For this review, use the dimensioned drawing (mm, ordinates from the lowest corner) and the shaded views. A direction names the side the tool comes from. Round coordinates to 2 decimals unless told otherwise and drop trailing zeros. Order: outer loops, then holes, each group sorted by start corner. A loop starts at its lowest first (then second) coordinate and runs counter-clockwise, first axis right, second up. Notation, with made-up numbers: (-6.75, 56) -> (39.25, 56) arc R19 cw to (39.25, 92) -> close; hole circle Ø11 at (64, -31). An arc over 180 degrees is marked (long way). Answer in a Markdown table with one row per item.
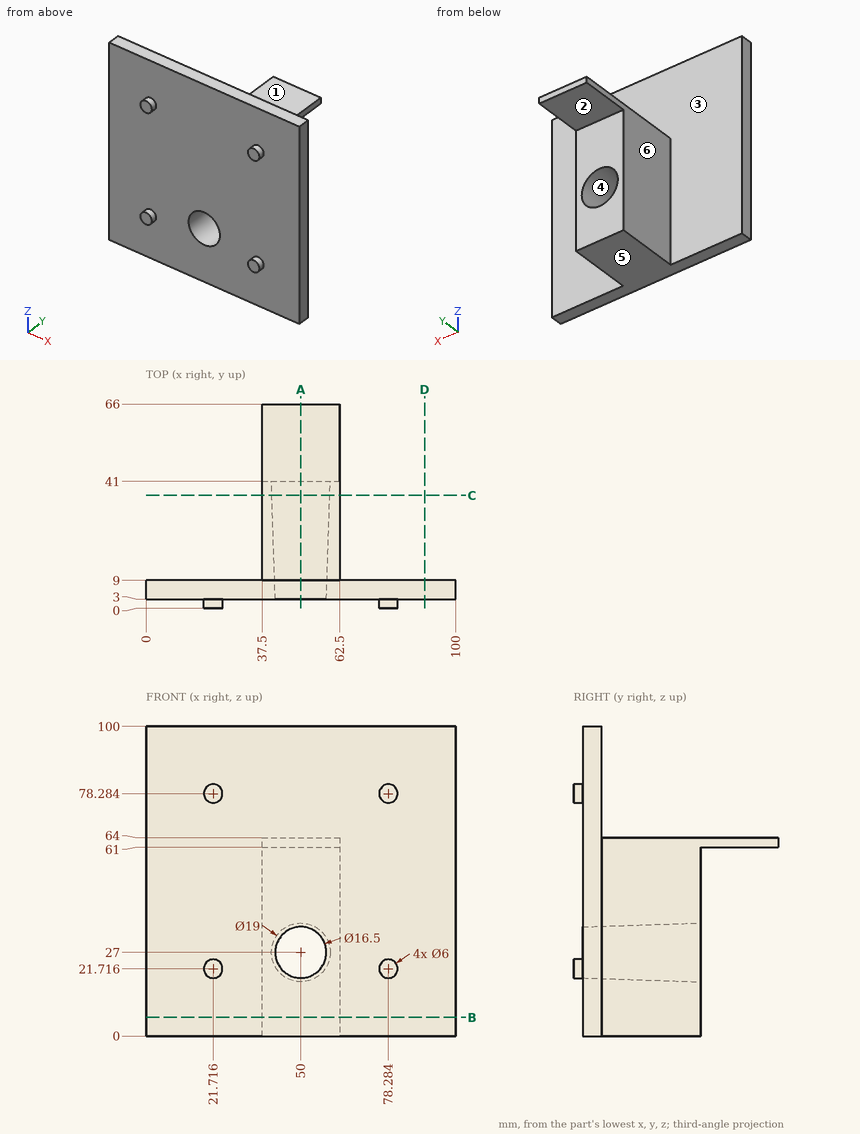
Q1. Take a section at D-D, the plane x = 90. Write out the cut boundary in (y, z).
Answer key:
| item | result |
|---|---|
| outline | (3, 0) -> (9, 0) -> (9, 100) -> (3, 100) -> close |
Q2. Tool access review of the marked faces 1, 2 and 3: name each direction out of +Z, -Z, +X, -X, +Y, -Y from which nothing blocks a thin tool from reaching the whole face with its end or side.
Answer key:
| item | result |
|---|---|
| face 1 | +Z, +X, -X, +Y |
| face 2 | -Z, +X, -X, +Y |
| face 3 | +Z, +Y |
Q3. To check wall thickness, follow probe 1 along Y at (x, z) = (27, 48); probe 2 along Y at (x, z) = (44, 50.5); probe 3 along X at (y, z) = (50.5, 63). State the ranges of each line that lie inside material, in increasing order.
Answer key:
| item | result |
|---|---|
| probe 1 | y = 3 to 9 |
| probe 2 | y = 3 to 41 |
| probe 3 | x = 37.5 to 62.5 |
Q4. Take a section at C-C, the plane y = 36.5. Write out the cut boundary in (x, z), then the cut area to 3 significant figures.
Answer key:
| item | result |
|---|---|
| outline | (37.5, 0) -> (62.5, 0) -> (62.5, 64) -> (37.5, 64) -> close; hole circle Ø18.7 at (50, 27) |
| area | 1,330 mm^2 |
Q5. Take a section at A-A, the plane x = 50. Write out the cut boundary in (y, z).
Answer key:
| item | result |
|---|---|
| outline | (3, 0) -> (41, 0) -> (41, 17.5) -> (3, 18.75) -> close; (3, 35.25) -> (41, 36.5) -> (41, 61) -> (66, 61) -> (66, 64) -> (9, 64) -> (9, 100) -> (3, 100) -> close |
Q6. Clearance check with flat-ended pins moving along their axes: pin 1 Ø7.5 at (x, y) = (53, 27) entering from +Z; pin 2 Ø2 at (x, z) = (20, 26) entering from -Y; pin 3 Ø5 at (x, z) = (19.5, 63) entering from +Y. State where each tip first meets the part, or that it passes through.
Answer key:
| item | result |
|---|---|
| pin 1 | stops at z = 64 |
| pin 2 | stops at y = 3 |
| pin 3 | stops at y = 9 |
Q7. Take a section at B-B, the plane z = 6. Write out the cut boundary in (x, y).
Answer key:
| item | result |
|---|---|
| outline | (0, 3) -> (100, 3) -> (100, 9) -> (62.5, 9) -> (62.5, 41) -> (37.5, 41) -> (37.5, 9) -> (0, 9) -> close |
Q8. The part is to be moulded in two halves that separate along Z. For the marked faces 4, 5 and 6, say which applies: +Z half, -Z half, draft (parallel to the pull), parting line (faces both ways), or undercut.
Answer key:
| item | result |
|---|---|
| face 4 | undercut |
| face 5 | -Z half |
| face 6 | draft |
